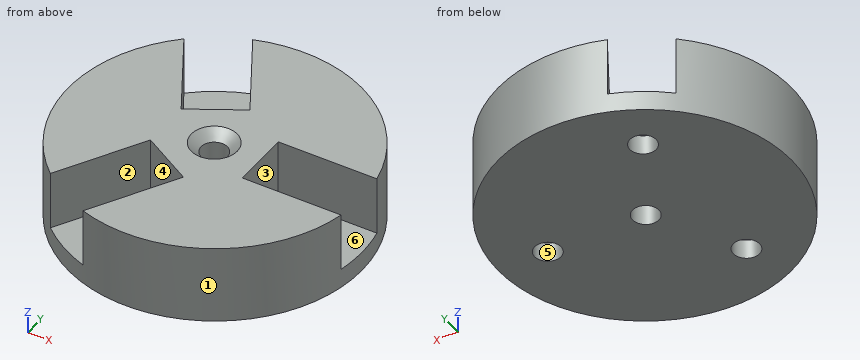
from build123d import *

# Parameters (mm, degrees)
SKETCH_R        = 15
SKETCH_R_2      = 1.35
PAD_DEPTH       = 8
POCKET_DEPTH    = 6
SKETCH002_R     = 1.35
POCKET001_DEPTH = 5
CHAMFER_SIZE    = 1


with BuildPart() as part:
    # Sketch → Pad (new body)
    with BuildSketch(Plane.XY):
        with Locations((0.085228, 0)):
            Circle(SKETCH_R)
        Circle(SKETCH_R_2, mode=Mode.SUBTRACT)
    extrude(amount=PAD_DEPTH)

    # Sketch001 → Pocket (cut)
    with BuildSketch(Plane.XY.offset(8)):
        with BuildLine():
            Line((4.698986, 3), (14.798986, 3))
            ThreePointArc((14.798986, -3), (15.1, 0), (14.798986, 3))
            Line((4.698986, -3), (14.798986, -3))
            Line((4.698986, 3), (4.698986, -3))
        make_face()
        with BuildLine():
            Line((-9.997569, 11.316298), (-4.947569, 2.569442))
            Line((-4.947569, 2.569442), (0.248583, 5.569442))
            Line((0.248583, 5.569442), (-4.801417, 14.316298))
            ThreePointArc((-4.801417, 14.316298), (-7.55, 13.076984), (-9.997569, 11.316298))
        make_face()
        with BuildLine():
            Line((-9.997569, -11.316298), (-4.947569, -2.569442))
            Line((-4.947569, -2.569442), (0.248583, -5.569442))
            Line((0.248583, -5.569442), (-4.801417, -14.316298))
            ThreePointArc((-9.997569, -11.316298), (-7.55, -13.076984), (-4.801417, -14.316298))
        make_face()
    extrude(amount=-POCKET_DEPTH, mode=Mode.SUBTRACT)

    # Sketch002 → Pocket001 (cut)
    with BuildSketch(Plane(origin=(0, 0, 0), x_dir=(1, 0, 0), z_dir=(0, 0, -1))):
        with Locations((10, 0)):
            Circle(SKETCH002_R)
        with Locations((-5, 8.660254)):
            Circle(SKETCH002_R)
        with Locations((-5, -8.660254)):
            Circle(SKETCH002_R)
    extrude(amount=-POCKET001_DEPTH, mode=Mode.SUBTRACT)

    # Chamfer
    chamfer_edges = [part.edges().sort_by_distance(p)[0] for p in [
        (-1.35, 0, 8),
    ]]
    chamfer(chamfer_edges, length=CHAMFER_SIZE)


solid = part.part
Can you work these out from the model? Positions are in its coordinate system, mm. Face numbers are marked on the shaded views. A direction names the side the tool comes from. Coordinates: 2 decimals unless noted, no trailing zeros. Write each loop counter-clockwise with the first axis right and the second up, starting at its lowest first coordinate (ties: lowest second). Pieces come first, ordered by that corner, then holes. Notation, with made-up numbers: (69, -17) -> (116, -17) arc R29 cw to (116, 13) -> close; hole circle Ø2 at (21, 79). An arc over 180 degrees is marked (long way). Write each question's results on one line, items separated by ' | '. Start each with the question number.
Q1. Imagine slicing it at D-D (y = -4.5). Write out the boundary of the cut face in (x, z).
Q2. On a 3-axis mill with a long thin cutter (end or side, diameter ignored), from which of +Z, -Z, +X, -X, +Y, -Y can I reach the whole of each face in a straight line? I mean the marked faces 4, 5 and 6. Say none if no direction works.
Q3. Imagine slicing it at A-A (y = 0). Write out the boundary of the cut face in (x, z).
Q4. We'd pull the mould along X, two halves only. Please class the marked faces 1, 2 and 3: +X half, -X half, draft (parallel to the pull), parting line (faces both ways), or undercut.
Q5. I'm going to push flat-ended pins straight in: pin 1 (2.5 mm diameter, centred on x = 0, y = 0, fed in from +Z); pin 2 (1 mm diameter, centred on x = -5, z = 3, fed in from +Y); pin 3 (5 mm diameter, centred on x = 9, y = 0, fed in from +Z); pin 4 (3 mm diameter, centred on y = 1, z = 5.5, fed in from +X). Where does each tip first touch, or does it pass through?
Q6. Imagine slicing it at C-C (x = -8.75). Write out the boundary of the cut face in (y, z), then the cut area to 3 significant figures.
Q7. If I drill on probe 1 along Y at (x, z) = (-4.25, 7); probe 2 along Y at (x, z) = (-5, 1.1); probe 3 along Y at (x, z) = (12.5, 6.5), over which ranges is the centre line in solid material (lowest first)?
Q8. Imagine slicing it at B-B (z = 5.5). Write out the boundary of the cut face in (x, y), then the cut area to 3 significant figures.
Taken from the geometry:
1) outline: (-14.22, 0) -> (14.39, 0) -> (14.39, 8) -> (-1.6, 8) -> (-1.6, 2) -> (-6.06, 2) -> (-6.06, 8) -> (-14.22, 8) -> close
2) face 4: +Z | face 5: +Z, -Z | face 6: +Z, +X
3) outline: (-14.91, 0) -> (-1.35, 0) -> (-1.35, 7) -> (-2.35, 8) -> (-14.91, 8) -> close; (1.35, 0) -> (8.65, 0) -> (8.65, 2) -> (4.7, 2) -> (4.7, 8) -> (2.35, 8) -> (1.35, 7) -> close; (11.35, 0) -> (15.09, 0) -> (15.09, 2) -> (11.35, 2) -> close
4) face 1: parting line | face 2: undercut | face 3: +X half
5) pin 1: passes through | pin 2: stops at y = 14.28 | pin 3: stops at z = 2 | pin 4: stops at x = 4.7
6) outline: (-12.12, 0) -> (12.12, 0) -> (12.12, 2) -> (9.16, 2) -> (9.16, 8) -> (-9.16, 8) -> (-9.16, 2) -> (-12.12, 2) -> close | area: 158 mm^2
7) probe 1: y = -14.36 to -13.36, -2.97 to 2.97, 13.36 to 14.36 | probe 2: y = -14.11 to -10.01, -7.31 to 7.31, 10.01 to 14.11 | probe 3: y = -8.42 to -3, 3 to 8.42
8) outline: (-9.92, -11.18) -> (-4.95, -2.57) -> (0.25, -5.57) -> (-4.74, -14.2) arc R15 ccw to (14.78, -3) -> (4.7, -3) -> (4.7, 3) -> (14.78, 3) arc R15 ccw to (-4.74, 14.2) -> (0.25, 5.57) -> (-4.95, 2.57) -> (-9.92, 11.18) arc R15 ccw to start; hole circle Ø2.7 at (0, 0) | area: 518 mm^2
